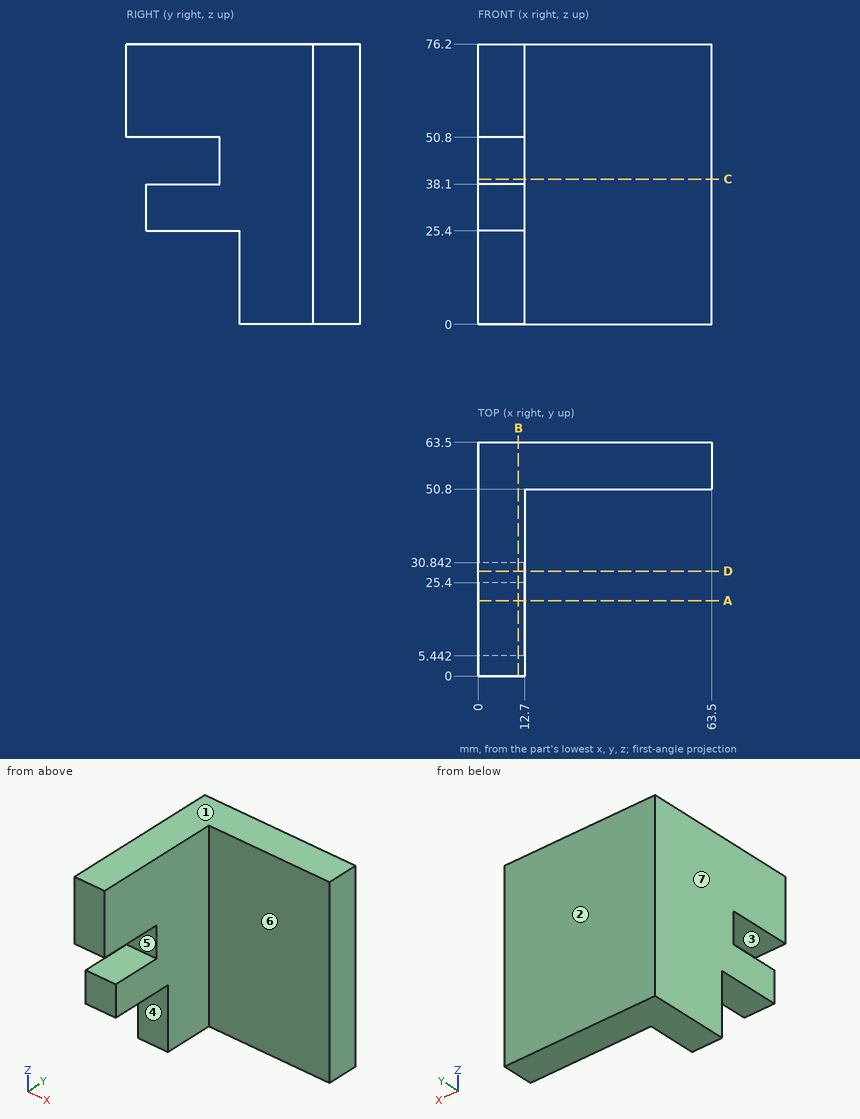
Input: dimensioned drawing with shaded views. Units: mm. Origin: part minimum x, y, z. A direction names the side the tool comes from. Coordinates: 2 decimals unless noted, no trailing zeros. Order: outer loops, then holes, each group sorted by start corner. A loop starts at its lowest first (then second) coordinate and runs counter-clockwise, first axis right, second up.
(1) First-contact query: pin 1 (14 mm diameter, centred on x = 9, y = 14, fed in from -Z); pin 2 (4 mm diameter, centred on x = 7, z = 12.5, fed in from -Y); pin 3 (14 mm diameter, centred on x = 4.5, z = 45, fed in from -Y); pin 4 (1 mm diameter, centred on x = 17, z = 64.5, fed in from -Y). Flat tips, straight axial feed; report the tip coordinate or a pass-through.
(2) Material intervals for probe 1 along Z at (x, y) = (4, 23); probe 2 along X at (y, z) = (32, 15); probe 3 along Y at (x, z) = (52, 57), sorted ascending.
(3) Access query for the marked faces 4, 5, 6 and 7. Directions: +Z, -Z, +X, -X, +Y, -Y. A direction counts if a zero-diameter tool reaches every point of the face in a straight line with its end or side. Return the directions, or none.
(4) Section query A-A (y = 20.5). Return the cut outline in (x, z).
(5) Section query D-D (y = 28.5). Return the cut outline in (x, z).
(6) Draft query along Z for the marked faces 1, 2 and 3. Return one class per face: pulls with the +Z half, pulls with the -Z half, needs draft (parallel to the pull), parting line crosses it, or undercut.
(7) Section query C-C (z = 39.5). Return the cut outline in (x, y), plus the area to 3 significant figures.
(8) Section query B-B (x = 11). Return the cut outline in (y, z), plus the area to 3 significant figures.
Solution:
1. pin 1: stops at z = 25.4
1. pin 2: stops at y = 30.84
1. pin 3: stops at y = 0
1. pin 4: stops at y = 50.8
2. probe 1: z = 25.4 to 38.1, 50.8 to 76.2
2. probe 2: x = 0 to 12.7
2. probe 3: y = 50.8 to 63.5
3. face 4: -Z, +X, -X, -Y
3. face 5: +X, -X, -Y
3. face 6: +Z, -Z, +X, -Y
3. face 7: +Z, -Z, -X, +Y, -Y
4. outline: (0, 25.4) - (12.7, 25.4) - (12.7, 38.1) - (0, 38.1) - close; (0, 50.8) - (12.7, 50.8) - (12.7, 76.2) - (0, 76.2) - close
5. outline: (0, 25.4) - (12.7, 25.4) - (12.7, 76.2) - (0, 76.2) - close
6. face 1: pulls with the +Z half
6. face 2: needs draft
6. face 3: undercut
7. outline: (0, 25.4) - (12.7, 25.4) - (12.7, 50.8) - (63.5, 50.8) - (63.5, 63.5) - (0, 63.5) - close
7. area: 1,130 mm2
8. outline: (0, 50.8) - (25.4, 50.8) - (25.4, 38.1) - (5.44, 38.1) - (5.44, 25.4) - (30.84, 25.4) - (30.84, 0) - (63.5, 0) - (63.5, 76.2) - (0, 76.2) - close
8. area: 3,660 mm2
